from build123d import *

# Parameters (mm, degrees)
F0_R     = 9
F0_R_2   = 5.5
F1_DEPTH = 35
F3_DEPTH = 25
F4_W     = 3
F4_H     = 26
F6_W     = 40
F6_H     = 26
F8_R     = 1


with BuildPart() as f1:
    # F0 (on Top) → F1 (new body)
    with BuildSketch(Plane.XY):
        Circle(F0_R)
        Circle(F0_R_2, mode=Mode.SUBTRACT)
    extrude(amount=F1_DEPTH)

    # F2 (on Right) → F3 (cut)
    with BuildSketch(Plane.YZ):
        with BuildLine():
            ThreePointArc((0, 4.5), (0.7071067812, 4.7928932188), (1, 5.5))
            Line((1, 5.5), (1, 29.5))
            ThreePointArc((1, 29.5), (0.7071067812, 30.2071067812), (0, 30.5))
            ThreePointArc((0, 30.5), (-0.7071067812, 30.2071067812), (-1, 29.5))
            Line((-1, 29.5), (-1, 5.5))
            ThreePointArc((-1, 5.5), (-0.7071067812, 4.7928932188), (0, 4.5))
        make_face()
    extrude(amount=-F3_DEPTH, mode=Mode.SUBTRACT)

    # F4 (on Right) → F7 section 0
    with BuildSketch(Plane.YZ):
        with Locations((0, 17.5)):
            Rectangle(F4_W, F4_H)
    # F6 (on offset) → F7 section 1
    with BuildSketch(Plane.YZ.offset(20)):
        with Locations((0, 17.5)):
            Rectangle(F6_W, F6_H)
    loft(mode=Mode.SUBTRACT)

    # F8
    f8_edges = [f1.edges().sort_by_distance(p)[0] for p in [
        (4.508802, -5.670642, 30.5),
        (4.508802, 5.670642, 30.5),
        (4.508802, 5.670642, 4.5),
        (4.508802, -5.670642, 4.5),
    ]]
    fillet(f8_edges, radius=F8_R)


solid = f1.part
Work out the finished part from the listing and answer in its coordinate system (mm). A direction names the side the tool comes from. Round coordinates to 2 decimals unless told otherwise and drop trailing zeros. Write each loop counter-clockwise with the first axis right and the second up, starting at its lowest first coordinate (ties: lowest second). Pieces come first, ordered by that corner, then holes.
1) Given pin 1 Ø3 at (x, z) = (-4.5, 9) entering from +Y; pin 2 Ø6.5 at (x, y) = (0, 0) entering from -Z; pin 3 Ø1 at (x, z) = (-1, 17.5) entering from +Y; pin 4 Ø1.5 at (x, z) = (-6, 12) entering from +Y, each flat-ended and moving along its own axis, determine where each tip first touches the part or whether it passes through.
2) A cutting plane is placed at B-B (x = 0). Give the vertices of the cut face in (y, z).
3) A tool of negligible diameter and unlimited length cuts with its end or side. For faces 1 (the cylindrical face through (-4.05, 3.72, 17.26)), 2 (the flat face through (-7, 1, 17)), 3 (the flat face through (4.53, 5.69, 17.33)), from which of +Z, -Z, +X, -X, +Y, -Y can it reach the whole face along a straight path? Write none if from no direction.
4) Straight lines are drawn through the part: line 1 (Z direction, x = 5.5, y = 1); line 2 (Y direction, x = 0, z = 10.5); line 3 (Y direction, x = -1.75, z = 32.5). For each, find the intervals that lie inside material, in ascending order.
5) The mould has two halves that part along Y. Classify faces 4 (the flat face through (-4, -4, 0)), 5 (the cylindrical face through (-6.633, 6.083, 17.255)), 6 (the flat face through (4.53, -5.69, 17.67)): pulls with the +Y half, pulls with the -Y half, needs draft (parallel to the pull), parting line crosses it, or undercut.
6) A cutting plane is placed at A-A (z = 7.5). Give the vertices of the cut face in (x, y), plus the area to 3 significant figures.
7) A cutting plane is placed at D-D (y = 0.5). Give the number of separate pieces and of enclosed holes in the cut face, plus the area to 3 significant figures.
8) A cutting plane is placed at C-C (x = -7). Give the vertices of the cut face in (y, z), plus the area to 3 significant figures.
Completed:
1. pin 1: stops at y = 8.49
1. pin 2: passes through
1. pin 3: stops at y = 8.99
1. pin 4: stops at y = 7.31
2. outline: (-9, 0) - (-5.5, 0) - (-5.5, 35) - (-9, 35) - close; (5.5, 0) - (9, 0) - (9, 35) - (5.5, 35) - close
3. face 1: +Z, -Z
3. face 2: +X, -X
3. face 3: +X
4. line 1: z = 0 to 4.5, 30.5 to 35
4. line 2: y = -9 to -5.5, 5.5 to 9
4. line 3: y = -8.83 to -5.21, 5.21 to 8.83
5. face 4: needs draft
5. face 5: parting line crosses it
5. face 6: undercut
6. outline: (-8.94, -1) arc R9 ccw to (5.81, -6.87) - (3.21, -4.47) arc R5.5 cw to (-5.41, -1) - close; (-8.94, 1) - (-5.41, 1) arc R5.5 cw to (3.21, 4.47) - (5.81, 6.87) arc R9 ccw to start
6. area: 107 mm2
7. separate pieces: 4
7. enclosed holes: 0
7. area: 64.1 mm2
8. outline: (-5.66, 0) - (5.66, 0) - (5.66, 35) - (-5.66, 35) - close; hole (-1, 5.5) arc R1 ccw to (1, 5.5) - (1, 29.5) arc R1 ccw to (-1, 29.5) - close
8. area: 345 mm2
